Read the model definition and answer for the solid it produces. Units are mm, in the model's axes. Face numbers are marked on the shaded views. A direction names the side the tool comes from. Round coordinates to 2 decimals unless told otherwise and drop trailing zeros. Order: outer loops, then holes, each group sorted by start corner. A loop starts at its lowest first (then second) coordinate and runs counter-clockwise, first axis right, second up. Notation, with made-up numbers: (81.5, 47.25) - (85.5, 47.25) arc R25 cw to (85.5, 67.25) - close; hole circle Ø4 at (72.25, -2.5). An arc over 180 degrees is marked (long way). Answer as a JSON object with one key per item and string values. Group by question number.
Q1. Consider line 1 (Y direction, x = 47.5, z = 37); line 2 (X direction, y = -29, z = 44); line 3 (Z direction, x = 19.5, y = -47). Determine where each line is inside the solid, lowest interval first.
Q2. A tool of negligible diameter and unlimited length cuts with its end or side. For the marked faces 1, 2, 3, 4 and 5, from which of +Z, -Z, +X, -X, +Y, -Y can it reach the whole face along a straight path? Write none if from no direction.
Q3. A cutting plane is placed at D-D on z = -33. Determine the outline of the cut face in (x, y).
Q4. Given pin 1 Ø15 at (x, z) = (-8, -25) entering from -Y; pin 2 Ø8 at (x, y) = (45.97, -8.78) entering from -Z; pin 3 Ø13 at (x, y) = (38.97, 16.22) entering from +Z; pin 4 Ø12 at (y, z) = (-26.5, -59) entering from +X, each flat-ended and moving along its own axis, determine where each tip first touches the part or whether it passes through.
Q5. A cutting plane is placed at B-B on y = -40. Determine the outline of the cut face in (x, z).
Q6. A cutting plane is placed at C-C on z = 27.5. Determine the outline of the cut face in (x, y), and give its area (3 significant figures).
Q7. A cutting plane is placed at A-A on x = -32.5. Determine the outline of the cut face in (y, z).
```python
from build123d import *

# Parameters (mm, degrees)
SKETCH_1_W             = 100
SKETCH_1_H             = 100
EXTRUDE_1_DEPTH        = 50
SKETCH_2_R             = 5
CUT_EXTRUDE_1_DEPTH    = 51
SKETCH_4_R             = 2.5
CUT_EXTRUDE_2_DEPTH    = 51
SKETCH_5_W             = 50
SKETCH_5_H             = 50
EXTRUDE_3_DEPTH        = 50
SKETCH_3_R             = 3.5
EXTRUDE_4_DEPTH        = 100
CHAMFER_4_SIZE         = 2
CHAMFER_4_SIZE2        = 2.383507185
CHAMFER_4_PART_2_SIZE  = 2
CHAMFER_4_PART_2_SIZE2 = 2.383507185
CHAMFER_4_PART_3_SIZE  = 2
CHAMFER_4_PART_3_SIZE2 = 2.383507185
CHAMFER_4_PART_4_SIZE  = 2
CHAMFER_4_PART_4_SIZE2 = 2.383507185


with BuildPart() as part:
    # 草图1 → 凸台-拉伸1 (new body)
    with BuildSketch(Plane.XY):
        with Locations((3.968253968, -18.783068783)):
            Rectangle(SKETCH_1_W, SKETCH_1_H)
    extrude(amount=EXTRUDE_1_DEPTH)

    # 草图2 → 切除-拉伸1 (cut, through all)
    with BuildSketch(Plane(origin=(0, 0, 0), x_dir=(-1, 0, 0), z_dir=(0, 0, -1))):
        with Locations((-38.968253968, 16.216931217)):
            Circle(SKETCH_2_R)
        with Locations((31.031746032, 16.216931217)):
            Circle(SKETCH_2_R)
        with Locations((-38.968253968, -53.783068783)):
            Circle(SKETCH_2_R)
        with Locations((31.031746032, -53.783068783)):
            Circle(SKETCH_2_R)
    extrude(amount=-CUT_EXTRUDE_1_DEPTH, mode=Mode.SUBTRACT)

    # 草图4 → 切除-拉伸2 (cut, through all)
    with BuildSketch(Plane(origin=(0, 0, 0), x_dir=(-1, 0, 0), z_dir=(0, 0, -1))):
        with Locations((-45.968253968, -8.783068783)):
            Circle(SKETCH_4_R)
        with Locations((-45.968253968, -28.783068783)):
            Circle(SKETCH_4_R)
    extrude(amount=-CUT_EXTRUDE_2_DEPTH, mode=Mode.SUBTRACT)

    # 草图5 → 凸台-拉伸3 (add)
    with BuildSketch(Plane(origin=(0, 0, 0), x_dir=(-1, 0, 0), z_dir=(0, 0, -1))):
        with Locations((-3.968253968, -18.783068783)):
            Rectangle(SKETCH_5_W, SKETCH_5_H)
    extrude(amount=EXTRUDE_3_DEPTH)

    # 草图3 → 凸台-拉伸4 (add)
    with BuildSketch(Plane(origin=(0, 0, 0), x_dir=(-1, 0, 0), z_dir=(0, 0, -1))):
        with Locations((-3.968253968, -3.783068783)):
            Circle(SKETCH_3_R)
        with Locations((-18.968253968, -18.783068783)):
            Circle(SKETCH_3_R)
        with Locations((-3.968253968, -33.783068783)):
            Circle(SKETCH_3_R)
        with Locations((11.031746032, -18.783068783)):
            Circle(SKETCH_3_R)
    extrude(amount=EXTRUDE_4_DEPTH)

    # 倒角4
    chamfer_4_edges = [part.edges().sort_by_distance(p)[0] for p in [
        (7.468253968, -3.783068783, -100),
    ]]
    chamfer_4_side = [part.faces().sort_by_distance(p)[0] for p in [
        (7.468253968, -3.783068783, -75),
    ]]
    chamfer(chamfer_4_edges, length=CHAMFER_4_SIZE, length2=CHAMFER_4_SIZE2, reference=chamfer_4_side[0])

    # 倒角4 part 2
    chamfer_4_part_2_edges = [part.edges().sort_by_distance(p)[0] for p in [
        (22.468253968, -18.783068783, -100),
    ]]
    chamfer_4_part_2_side = [part.faces().sort_by_distance(p)[0] for p in [
        (22.468253968, -18.783068783, -75),
    ]]
    chamfer(chamfer_4_part_2_edges, length=CHAMFER_4_PART_2_SIZE, length2=CHAMFER_4_PART_2_SIZE2, reference=chamfer_4_part_2_side[0])

    # 倒角4 part 3
    chamfer_4_part_3_edges = [part.edges().sort_by_distance(p)[0] for p in [
        (7.468253968, -33.783068783, -100),
    ]]
    chamfer_4_part_3_side = [part.faces().sort_by_distance(p)[0] for p in [
        (7.468253968, -33.783068783, -75),
    ]]
    chamfer(chamfer_4_part_3_edges, length=CHAMFER_4_PART_3_SIZE, length2=CHAMFER_4_PART_3_SIZE2, reference=chamfer_4_part_3_side[0])

    # 倒角4 part 4
    chamfer_4_part_4_edges = [part.edges().sort_by_distance(p)[0] for p in [
        (-7.531746032, -18.783068783, -100),
    ]]
    chamfer_4_part_4_side = [part.faces().sort_by_distance(p)[0] for p in [
        (-7.531746032, -18.783068783, -75),
    ]]
    chamfer(chamfer_4_part_4_edges, length=CHAMFER_4_PART_4_SIZE, length2=CHAMFER_4_PART_4_SIZE2, reference=chamfer_4_part_4_side[0])


solid = part.part
```
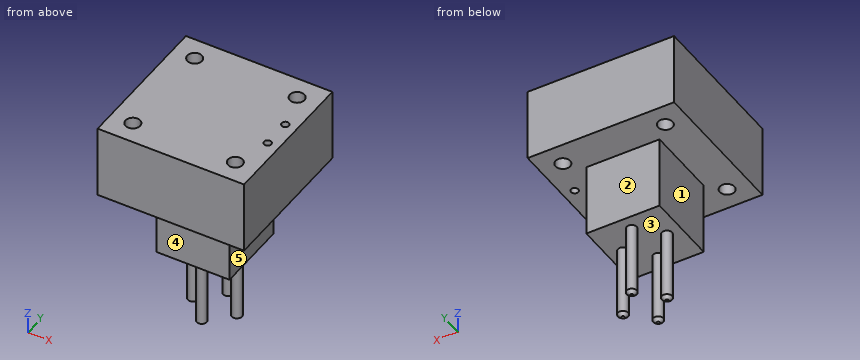
Result set:
{
 "1": {"line 1": "y = -68.78 to -30.76, -26.81 to -10.76, -6.81 to 31.22", "line 2": "x = -46.03 to 43.48, 48.46 to 53.97", "line 3": "z = 0 to 50"},
 "2": {"face 1": "-Z, -X, +Y, -Y", "face 2": "-Z, +X, -X, +Y", "face 3": "-Z", "face 4": "-Z, +X, -X, -Y", "face 5": "-Z, +X, +Y, -Y"},
 "3": {"outline": "(-21.03, -43.78) - (28.97, -43.78) - (28.97, 6.22) - (-21.03, 6.22) - close"},
 "4": {"pin 1": "stops at y = -43.78", "pin 2": "stops at z = 0", "pin 3": "stops at z = 50", "pin 4": "stops at x = 22.02"},
 "5": {"outline": "(-46.03, 0) - (-21.03, 0) - (-21.03, -50) - (28.97, -50) - (28.97, 0) - (53.97, 0) - (53.97, 50) - (-46.03, 50) - close"},
 "6": {"outline": "(-46.03, -68.78) - (53.97, -68.78) - (53.97, 31.22) - (-46.03, 31.22) - close; hole circle Ø10 at (-31.03, -53.78); hole circle Ø10 at (-31.03, 16.22); hole circle Ø10 at (38.97, -53.78); hole circle Ø10 at (38.97, 16.22); hole circle Ø5 at (45.97, -28.78); hole circle Ø5 at (45.97, -8.78)", "area": "9,650 mm²"},
 "7": {"outline": "(-68.78, 0) - (-58.56, 0) - (-58.56, 50) - (-68.78, 50) - close; (-49, 0) - (11.44, 0) - (11.44, 50) - (-49, 50) - close; (21, 0) - (31.22, 0) - (31.22, 50) - (21, 50) - close"}
}
